Here's the drawing with two shaded views (mm, measured from the low corner). I have some questions. Give positions to 0.01 mm unless a question says otherwise; leave off trailing zeros. Loops run counter-clockwise (first coordinate to the right, second up) from the corner with the lowest first, then second, coordinate; pieces in that order, holes last. Notation, with made-up numbers: (24, 18.25) -> (52, 18.25) arc R29 ccw to (52, 53.25) -> close; hole circle Ø9 at (71.25, -20). An arc over 180 degrees is marked (long way). Put each result on its own line as item: value.
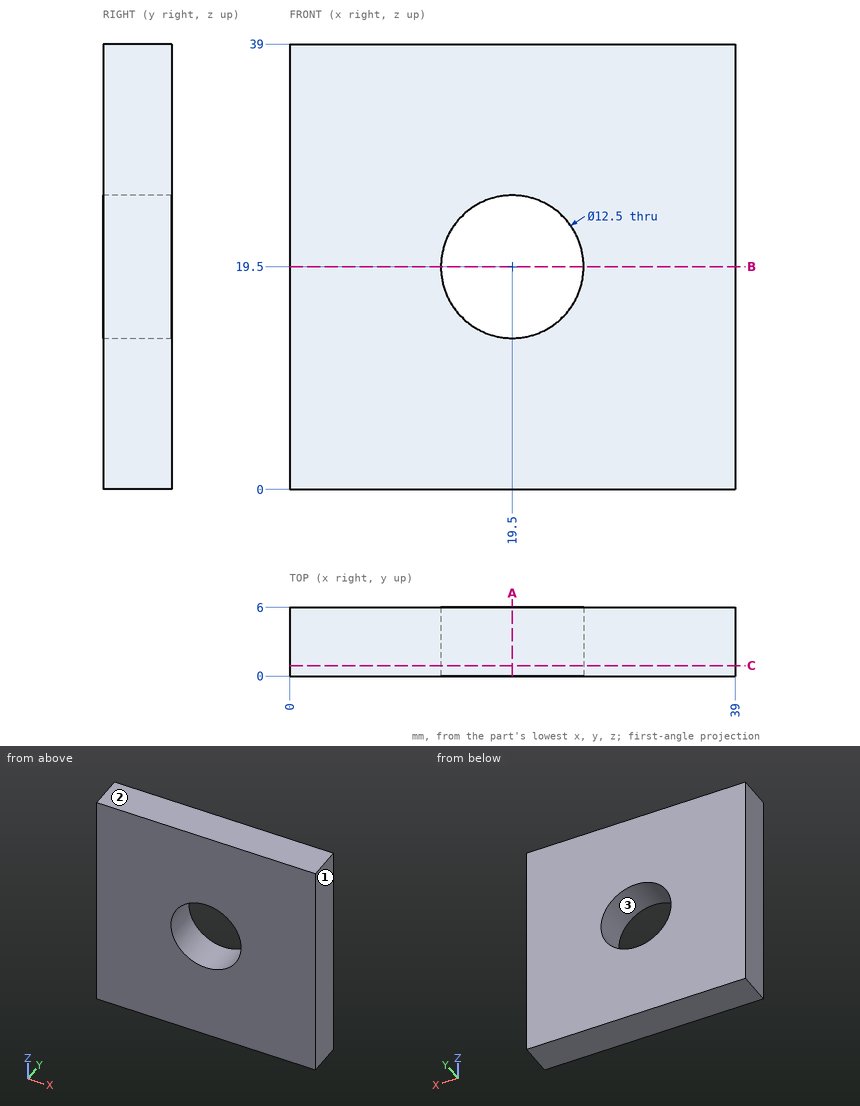
1. If we section it at A-A (x = 19.5): List the corners of the cut face in (y, z) for me.
Recorded:
outline: (0, 0) -> (6, 0) -> (6, 13.25) -> (0, 13.25) -> close; (0, 25.75) -> (6, 25.75) -> (6, 39) -> (0, 39) -> close
2. If we section it at B-B (z = 19.5): List the corners of the cut face in (x, y) for me, then the cut area to 3 significant figures.
Recorded:
outline: (0, 0) -> (13.25, 0) -> (13.25, 6) -> (0, 6) -> close; (25.75, 0) -> (39, 0) -> (39, 6) -> (25.75, 6) -> close
area: 159 mm^2
3. If we section it at C-C (y = 0.9): List the corners of the cut face in (x, z) for me, then the cut area to 3 significant figures.
Recorded:
outline: (0, 0) -> (39, 0) -> (39, 39) -> (0, 39) -> close; hole circle Ø12.5 at (19.5, 19.5)
area: 1,400 mm^2
4. I need wall thicknesses on line 1 (X direction, y = 4.3, z = 19.5); line 2 (X direction, y = 4.35, z = 18). Which ranges of each line are inside material? Lowest first, please.
Recorded:
line 1: x = 0 to 13.25, 25.75 to 39
line 2: x = 0 to 13.43, 25.57 to 39
5. Thinking about a two-plate mould opening in X: for the marked faces 1, 2 and 3, which applies, pulls with the +X half, pulls with the -X half, needs draft (parallel to the pull), parting line crosses it, or undercut?
Recorded:
face 1: pulls with the +X half
face 2: needs draft
face 3: undercut
